Design review of the part built by this model. Coordinates are the model's own, in mm. A direction names the side the tool comes from. Coordinates: 2 decimals unless noted, no trailing zeros. Loops run counter-clockwise (first coordinate to the right, second up) from the corner with the lowest first, then second, coordinate; pieces in that order, holes last. Notation, with made-up numbers: (-14, 21.5) -> (-2, 21.5) arc R23 cw to (-2, 45.5) -> close; hole circle Ø1 at (35.5, 50). An arc over 180 degrees is marked (long way). Answer in a Markdown table with one row per item.
```python
from build123d import *

# Parameters (mm, degrees)
SKETCH1_W                      = 185
SKETCH1_H                      = 44.2
BOSS_EXTRUDE1_DEPTH            = 11.25
SKETCH2_W                      = 25
SKETCH2_H                      = 44.2
CUT_EXTRUDE1_DEPTH             = 8.25
FILLET1_R                      = 5
CUT_EXTRUDE2_DEPTH             = 15.2
LPATTERN1_COUNT                = 9
LPATTERN1_PITCH                = 17.2
SKETCH4_W                      = 4.5
SKETCH4_H                      = 44.2
BOSS_EXTRUDE2_DEPTH            = 35
CBORE_FOR_M3_SHCS1_D           = 3.4
CBORE_FOR_M3_SHCS1_DEPTH       = 10.1
CBORE_FOR_M3_SHCS1_CBORE_D     = 6.5
CBORE_FOR_M3_SHCS1_CBORE_DEPTH = 3
CBORE_FOR_M3_SHCS1_TIP         = 1.021463052
CUT_EXTRUDE3_DEPTH             = 35
FILLET2_R                      = 1
FILLET3_R                      = 1


with BuildPart() as part:
    # Sketch1 → Boss-Extrude1 (new body)
    with BuildSketch(Plane.XY):
        Rectangle(SKETCH1_W, SKETCH1_H)
    extrude(amount=BOSS_EXTRUDE1_DEPTH)

    # Sketch2 → Cut-Extrude1 (cut)
    with BuildSketch(Plane.XY.offset(11.25)):
        with Locations((-80, 0)):
            Rectangle(SKETCH2_W, SKETCH2_H)
    extrude(amount=-CUT_EXTRUDE1_DEPTH, mode=Mode.SUBTRACT)

    # Fillet1
    fillet1_edges = [part.edges().sort_by_distance(p)[0] for p in [
        (-67.5, 0, 3),
    ]]
    fillet(fillet1_edges, radius=FILLET1_R)

    # Sketch3 → Cut-Extrude2 (cut)
    with BuildSketch(Plane.ZY.offset(66)):
        Polygon((0, 8.85), (1.15, 8.85), (1.15, 10.35), (8.25, 10.35), (8.25, 8.85), (11.25, 8.85), (11.25, -10.6), (8.25, -10.6), (8.25, -12.1), (1.15, -12.1), (1.15, -10.545741226), (0, -7.36), align=None)
    cut_extrude2 = extrude(amount=-CUT_EXTRUDE2_DEPTH, mode=Mode.SUBTRACT)

    # LPattern1: Cut-Extrude2 ×9
    with Locations(*[(i * LPATTERN1_PITCH, 0, 0) for i in range(1, LPATTERN1_COUNT)]):
        add(cut_extrude2, mode=Mode.SUBTRACT)

    # Sketch4 → Boss-Extrude2 (add)
    with BuildSketch(Plane.XY.offset(11.25)):
        with Locations((90.25, 0)):
            Rectangle(SKETCH4_W, SKETCH4_H)
    extrude(amount=BOSS_EXTRUDE2_DEPTH)

    # CBORE for M3 SHCS1
    with Locations(Plane.ZY.offset(-86.8)):
        with Locations((17, 9.6), (37, 9.6), (17, -10.4), (37, -10.4)):
            CounterBoreHole(CBORE_FOR_M3_SHCS1_D / 2, CBORE_FOR_M3_SHCS1_CBORE_D / 2, CBORE_FOR_M3_SHCS1_CBORE_DEPTH, depth=CBORE_FOR_M3_SHCS1_DEPTH)
            with Locations((0, 0, -(CBORE_FOR_M3_SHCS1_DEPTH + CBORE_FOR_M3_SHCS1_TIP / 2))):  # 118° drill point
                Cone(0, CBORE_FOR_M3_SHCS1_D / 2, CBORE_FOR_M3_SHCS1_TIP, mode=Mode.SUBTRACT)

    # Sketch10 → Cut-Extrude3 (cut)
    with BuildSketch(Plane(origin=(0, 0, 0), x_dir=(-1, 0, 0), z_dir=(0, 0, -1))):
        with BuildLine():
            Line((76.7, 18.6), (84.7, 18.6))
            ThreePointArc((84.7, 18.6), (87.4, 15.9), (84.7, 13.2))
            Line((84.7, 13.2), (76.7, 13.2))
            ThreePointArc((76.7, 13.2), (74, 15.9), (76.7, 18.6))
        make_face()
        with BuildLine():
            Line((76.7, -13.2), (84.7, -13.2))
            ThreePointArc((84.7, -13.2), (87.4, -15.9), (84.7, -18.6))
            Line((84.7, -18.6), (76.7, -18.6))
            ThreePointArc((76.7, -18.6), (74, -15.9), (76.7, -13.2))
        make_face()
    extrude(amount=-CUT_EXTRUDE3_DEPTH, mode=Mode.SUBTRACT)

    # Fillet2
    fillet2_edges = [part.edges().sort_by_distance(p)[0] for p in [
        (-41.2, 8.85, 11.25),
        (-41.2, -10.6, 11.25),
        (-24, 8.85, 11.25),
        (-24, -10.6, 11.25),
        (-6.8, 8.85, 11.25),
        (-6.8, -10.6, 11.25),
        (10.4, 8.85, 11.25),
        (10.4, -10.6, 11.25),
        (27.6, 8.85, 11.25),
        (27.6, -10.6, 11.25),
        (44.8, 8.85, 11.25),
        (44.8, -10.6, 11.25),
        (62, 8.85, 11.25),
        (62, -10.6, 11.25),
        (79.2, 8.85, 11.25),
        (79.2, -10.6, 11.25),
        (-58.4, 8.85, 11.25),
        (-58.4, -10.6, 11.25),
    ]]
    fillet(fillet2_edges, radius=FILLET2_R)

    # Fillet3
    fillet3_edges = [part.edges().sort_by_distance(p)[0] for p in [
        (0, -22.1, 0),
        (-92.5, 0, 0),
        (0, 22.1, 0),
    ]]
    fillet(fillet3_edges, radius=FILLET3_R)


solid = part.part
```
(1) Tool access review of faces 1 (the flat face through (89.8, -12, 18)), 2 (the flat face through (79.094, -8.975, 0.583)), 3 (the flat face through (-67.5, 0, 10)): name each direction out of +Z, -Z, +X, -X, +Y, -Y from which nothing blocks a thin tool from reaching the whole face with its end or side.
Evaluation:
| item | result |
|---|---|
| face 1 | -X |
| face 2 | +Z |
| face 3 | +Z, -X, +Y, -Y |
(2) Draft analysis for pull direction Z (two halves, no side actions). For faces 4 (the flat face through (-83, 0, 3)), 5 (the cylindrical face through (-87.4, 16, 1.5)), 6 (the cylindrical face through (91.2, -11.9, 16.2)), state which applies: pulls with the +Z half, pulls with the -Z half, needs draft (parallel to the pull), parting line crosses it, or undercut.
Evaluation:
| item | result |
|---|---|
| face 4 | pulls with the +Z half |
| face 5 | needs draft |
| face 6 | undercut |
(3) To check wall thickness, follow probe 1 along Y at (x, z) = (91.4, 37); probe 2 along Z at (x, y) = (89, -10); probe 3 along Y at (x, z) = (-30, 6). State the ranges of each line that lie inside material, in increasing order.
Evaluation:
| item | result |
|---|---|
| probe 1 | y = -22.1 to -12.1, -8.7 to 7.9, 11.3 to 22.1 |
| probe 2 | z = 0 to 13.77, 20.23 to 33.77, 40.23 to 46.25 |
| probe 3 | y = -22.1 to -12.1, 10.35 to 22.1 |
(4) For pin 1 (1.2 mm diameter, centred on x = -56.5, y = -11, fed in from +Z); pin 2 (3 mm diameter, centred on x = -4, y = -7.5, fed in from +Z); pin 3 (6 mm diameter, centred on x = 46.5, z = 17, fed in from -Y); pin 4 (6 mm diameter, centred on y = -1, z = 25, fed in from -X), all flat-tipped, find the tip position at first contact; note any pin that passes through.
Evaluation:
| item | result |
|---|---|
| pin 1 | stops at z = 11.25 |
| pin 2 | stops at z = 0.59 |
| pin 3 | passes through |
| pin 4 | stops at x = 88 |
(5) Take a section at C-C on z = 17. Give the boundary of the cut face in (x, y).
Evaluation:
| item | result |
|---|---|
| outline | (88, -22.1) -> (92.5, -22.1) -> (92.5, -12.1) -> (89.8, -12.1) -> (89.8, -13.65) -> (88, -13.65) -> close; (88, -7.15) -> (89.8, -7.15) -> (89.8, -8.7) -> (92.5, -8.7) -> (92.5, 7.9) -> (89.8, 7.9) -> (89.8, 6.35) -> (88, 6.35) -> close; (88, 12.85) -> (89.8, 12.85) -> (89.8, 11.3) -> (92.5, 11.3) -> (92.5, 22.1) -> (88, 22.1) -> close |
(6) Take a section at B-B on y = 15.9. Give the boundary of the cut face in (x, z).
Evaluation:
| item | result |
|---|---|
| outline | (-92.5, 1) arc R1 ccw to (-91.5, 0) -> (-87.4, 0) -> (-87.4, 3) -> (-92.5, 3) -> close; (-74, 0) -> (92.5, 0) -> (92.5, 46.25) -> (88, 46.25) -> (88, 11.25) -> (-67.5, 11.25) -> (-67.5, 8) arc R5 cw to (-72.5, 3) -> (-74, 3) -> close |
(7) Take a section at A-A on x = 48. Give the boundary of the cut face in (y, z).
Evaluation:
| item | result |
|---|---|
| outline | (-22.1, 1) arc R1 ccw to (-21.1, 0) -> (-7.36, 0) -> (-10.55, 1.15) -> (-12.1, 1.15) -> (-12.1, 8.25) -> (-10.6, 8.25) -> (-10.6, 10.25) arc R1 ccw to (-11.6, 11.25) -> (-22.1, 11.25) -> close; (8.85, 0) -> (21.1, 0) arc R1 ccw to (22.1, 1) -> (22.1, 11.25) -> (9.85, 11.25) arc R1 ccw to (8.85, 10.25) -> (8.85, 8.25) -> (10.35, 8.25) -> (10.35, 1.15) -> (8.85, 1.15) -> close |
(8) Take a section at D-D on y = -1.5. Count the separate pieces of the cut face and the enclosed holes in it, and give its area (3 significant figures).
Evaluation:
| item | result |
|---|---|
| separate pieces | 10 |
| enclosed holes | 0 |
| area | 499 mm² |
